Study the drawing (mm; zero at the part's minimum x, y, z) and answer. A direction names the side the tool comes from. Coordinates: 2 decimals unless noted, no trailing zeros. Write each loop counter-clockwise with the first axis right and the second up, starting at its lowest first coordinate (ties: lowest second). Pieces come first, ordered by that corner, then holes. Notation, with made-up numbers: (29.5, 25) -> (76.5, 25) arc R14 ccw to (76.5, 48) -> close; hole circle Ø4 at (27.5, 79). An arc over 180 degrees is marked (long way). Write item = value, one per line. Start each with the question number.
1) Find the intervals of material crossed by line 1 along Y through (x, z) = (8, 2.05); line 2 along Z through (x, y) = (54, 120); line 3 along X through (y, z) = (110, 0.9), in increasing order. Write a range as from..to.
2) A tool of negligible diameter and unlimited length cuts with its end or side. For the marked faces 1 and 2, from which of +Z, -Z, +X, -X, +Y, -Y can it reach the whole face along a straight path? Write none if from no direction.
3) Section D-D (z = 12) is taken. Determine the outline of the cut face in (x, y).
4) Section B-B (x = 20.5) is taken. Determine the outline of the cut face in (y, z).
5) Section C-C (y = 30) is taken. Determine the outline of the cut face in (x, z), plus the area to 3 significant figures.
6) Flat-ended cylindrical pins translate along their axes: pin 1 Ø5 at (x, y) = (15, 93.5) entering from -Z; pin 2 Ø3 at (x, y) = (58, 97) entering from +Z; pin 3 Ø1 at (y, z) = (41, 11.5) entering from +X; pin 4 Ø3.5 at (x, y) = (8, 5) entering from +Z. Find the tip coordinate at first contact, or state that the pin passes through.
7) Section A-A (y = 110) is taken. Determine the outline of the cut face in (x, z).
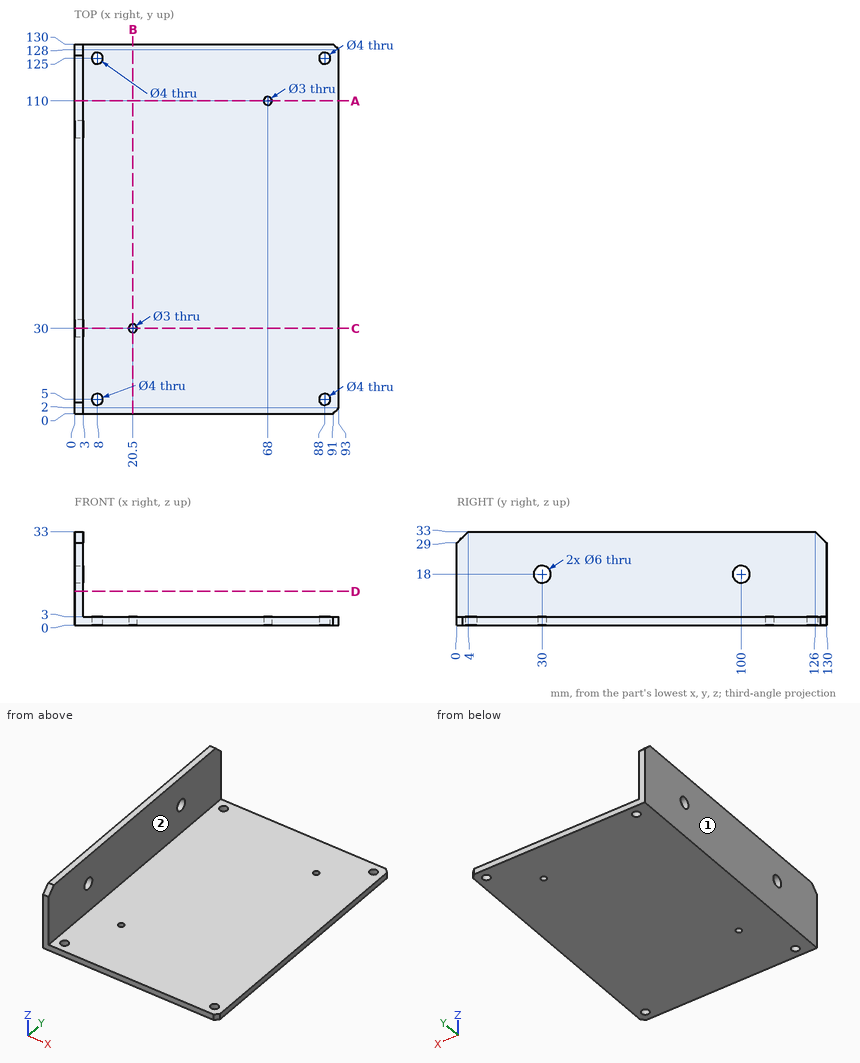
Answer key:
q1.line_1 = 0..3, 7..123, 127..130
q1.line_2 = 0..3
q1.line_3 = 0..66.5, 69.5..93
q2.face_1 = +Z, -Z, -X, +Y, -Y
q2.face_2 = +Z, +X, +Y, -Y
q3.outline = (0, 0) -> (3, 0) -> (3, 130) -> (0, 130) -> close
q4.outline = (0, 0) -> (28.5, 0) -> (28.5, 3) -> (0, 3) -> close; (31.5, 0) -> (130, 0) -> (130, 3) -> (31.5, 3) -> close
q5.outline = (0, 0) -> (19, 0) -> (19, 3) -> (3, 3) -> (3, 15) -> (0, 15) -> close; (0, 21) -> (3, 21) -> (3, 33) -> (0, 33) -> close; (22, 0) -> (93, 0) -> (93, 3) -> (22, 3) -> close
q5.area = 342 mm^2
q6.pin_1 = 0
q6.pin_2 = 3
q6.pin_3 = 3
q6.pin_4 = through
q7.outline = (0, 0) -> (66.5, 0) -> (66.5, 3) -> (3, 3) -> (3, 33) -> (0, 33) -> close; (69.5, 0) -> (93, 0) -> (93, 3) -> (69.5, 3) -> close
